Geometry: final body of the model. Coordinates: model frame, mm. A direction names the side the tool comes from. Round coordinates to 2 decimals unless told otherwise and drop trailing zeros. Write each loop counter-clockwise with the first axis right and the second up, starting at its lowest first coordinate (ties: lowest second). Pieces come first, ordered by that corner, then holes. Notation, with made-up numbers: (53, 51.5) -> (84, 51.5) arc R10 ccw to (84, 65.5) -> close; hole circle Ø10 at (84, 10.5). An arc over 180 degrees is marked (long way). One line per item, written item: value. Start each with the question number.
from build123d import *

# Parameters (mm, degrees)
SKETCH_1_W          = 15
SKETCH_1_H          = 15
SKETCH_1_W_2        = 13
SKETCH_1_H_2        = 13
EXTRUDE_1_DEPTH     = 570
SKETCH_2_R          = 1.45
CUT_EXTRUDE_1_DEPTH = 571.246657158
SKETCH_3_R          = 1.45
CUT_EXTRUDE_2_DEPTH = 571.246657158


with BuildPart() as part:
    # 草图1 → 凸台-拉伸1 (new body)
    with BuildSketch(Plane(origin=(0, 0, 0), x_dir=(0, 0, -1), z_dir=(1, 0, 0))):
        Rectangle(SKETCH_1_W, SKETCH_1_H)
        Rectangle(SKETCH_1_W_2, SKETCH_1_H_2, mode=Mode.SUBTRACT)
    extrude(amount=EXTRUDE_1_DEPTH)

    # 草图2 → 切除-拉伸1 (cut, through all)
    with BuildSketch(Plane(origin=(0, 7.5, 0), x_dir=(1, 0, 0), z_dir=(0, 1, 0))):
        with Locations(Location((561, 0, 0), (0, 0, 270))):
            Circle(SKETCH_2_R)
        with Locations(Location((551, 0, 0), (0, 0, 270))):
            Circle(SKETCH_2_R)
        with Locations(Location((297.5, 0, 0), (0, 0, 270))):
            Circle(SKETCH_2_R)
        with Locations(Location((272.5, 0, 0), (0, 0, 270))):
            Circle(SKETCH_2_R)
        with Locations(Location((24, 0, 0), (0, 0, 270))):
            Circle(SKETCH_2_R)
        with Locations(Location((14, 0, 0), (0, 0, 270))):
            Circle(SKETCH_2_R)
        with Locations(Location((97.5, 0, 0), (0, 0, 270))):
            Circle(SKETCH_2_R)
        with Locations(Location((77.5, 0, 0), (0, 0, 270))):
            Circle(SKETCH_2_R)
        with Locations(Location((57.5, 0, 0), (0, 0, 270))):
            Circle(SKETCH_2_R)
        with Locations(Location((472.5, 0, 0), (0, 0, 270))):
            Circle(SKETCH_2_R)
        with Locations(Location((492.5, 0, 0), (0, 0, 270))):
            Circle(SKETCH_2_R)
        with Locations(Location((512.5, 0, 0), (0, 0, 270))):
            Circle(SKETCH_2_R)
        with Locations(Location((346.5, 0, 0), (0, 0, 270))):
            Circle(SKETCH_2_R)
        with Locations(Location((326.5, 0, 0), (0, 0, 270))):
            Circle(SKETCH_2_R)
        with Locations(Location((248.5, 0, 0), (0, 0, 270))):
            Circle(SKETCH_2_R)
        with Locations(Location((225, 0, 0), (0, 0, 270))):
            Circle(SKETCH_2_R)
    extrude(amount=-CUT_EXTRUDE_1_DEPTH, mode=Mode.SUBTRACT)

    # 草图3 → 切除-拉伸2 (cut, through all)
    with BuildSketch(Plane.XY.offset(7.5)):
        with Locations((440, 0)):
            Circle(SKETCH_3_R)
        with Locations((405, 0)):
            Circle(SKETCH_3_R)
        with Locations((165, 0)):
            Circle(SKETCH_3_R)
        with Locations((130, 0)):
            Circle(SKETCH_3_R)
        with Locations((19, 0)):
            Circle(SKETCH_3_R)
        with Locations((9, 0)):
            Circle(SKETCH_3_R)
        with Locations((556, 0)):
            Circle(SKETCH_3_R)
        with Locations((546, 0)):
            Circle(SKETCH_3_R)
    extrude(amount=-CUT_EXTRUDE_2_DEPTH, mode=Mode.SUBTRACT)


solid = part.part
(1) Section query B-B (x = 422.5). Output: boundary loops of the cut face in (y, z), and give its area (3 significant figures).
(2) Pull-direction query (Z, two-part tool) for faces 3 (the face through (281, 0, -7.5)), 4 (the face through (281, 6.5, 0)), 5 (the face through (0, 0, 7)), 6 (the face through (281, 0, 6.5)); classes: pulls with the +Z half, pulls with the -Z half, needs draft (parallel to the pull), parting line crosses it, or undercut.
(3) Pin query (flat end, axial travel): pin 1 (2.5 mm diameter, centred on x = 57.5, z = 0, fed in from -Y). Return the tip coordinate at first contact, or that it passes through.
(4) Section query A-A (z = 4.25). Output: boundary loops of the cut face in (x, y).
(5) Line query: probe 1 along Z at (x, y) = (326.5, 7.15); probe 2 along Z at (x, y) = (270, 2.25). Output: solid intervals per line, ascending.
(6) Set-up query: faces 1 (the face through (281, 7.5, 0)), 2 (the face through (281, 0, -6.5)). Return all of +Z, -Z, +X, -X, +Y, -Y with unobstructed straight access to the full face (end or side cutting, diameter ignored); none if empty.
Results list:
1. outline: (-7.5, -7.5) -> (7.5, -7.5) -> (7.5, 7.5) -> (-7.5, 7.5) -> close; hole (-6.5, -6.5) -> (6.5, -6.5) -> (6.5, 6.5) -> (-6.5, 6.5) -> close
1. area: 56.0 mm^2
2. face 3: pulls with the -Z half
2. face 4: undercut
2. face 5: needs draft
2. face 6: undercut
3. pin 1: passes through
4. outline: (0, -7.5) -> (570, -7.5) -> (570, -6.5) -> (0, -6.5) -> close; (0, 6.5) -> (570, 6.5) -> (570, 7.5) -> (0, 7.5) -> close
5. probe 1: z = -7.5 to -1.45, 1.45 to 7.5
5. probe 2: z = -7.5 to -6.5, 6.5 to 7.5
6. face 1: +Z, -Z, +X, -X, +Y
6. face 2: +X, -X
